Autodesk Inventor part; units mm, degrees
ref_plane "YZ Plane" through (0, 0, 0) normal (1, 0, 0) x (0, 1, 0)
ref_plane "XZ Plane" through (0, 0, 0) normal (0, 1, 0) x (-1, 0, 0)
ref_plane "XY Plane" through (0, 0, 0) normal (0, 0, 1) x (1, 0, 0)
sketch "Sketch1" plane through (0, 0, 0) normal (0, 0, 1) x (1, 0, 0)
  line L0 (-65, 5) -> (65, 5)
  line L1 (65, 5) -> (65, -5)
  line L2 (65, -5) -> (-65, -5)
  line L3 (-65, -5) -> (-65, 5)
  circle A0 centre (0, 0) radius 2.4
  circle A1 centre (-54, 0) radius 2.4
  circle A2 centre (-27, 0) radius 2.4
  circle A3 centre (27, 0) radius 2.4
  circle A4 centre (54, 0) radius 2.4
  line L4 (-65, 0) -> (65, 0) construction
  point P0 (0, 5)
  dimension "d0" = 130
  dimension "d1" = 10
  dimension "d2" = 4.8
  dimension "d3" = 4.8
  dimension "d4" = 4.8
  dimension "d5" = 4.8
  dimension "d6" = 4.8
  dimension "d9" = 27
  dimension "d10" = 27
  dimension "d11" = 27
  dimension "d12" = 27
extrude "Plate1" add sketch "Sketch1" along normal blind 0.5
sketch "Sketch2" plane through (64.5, -5, 0.5) normal (1, 0, 0) x (0, 1, 0)
  line L0 (10, 0) -> (0, 0)
  line L1 (0, 0) -> (0, -5)
  line L2 (0, -5) -> (10, -5)
  line L3 (10, -5) -> (10, 0)
edge flange "Flange1" height 5 angle 90 thickness 0.5 bend radius 0.5 thickness toward (1, 0, 0) relief tear relief width 0.5 relief depth 0.25 corner gap 0.5 corner form 0 edges at (65, 0, 0) (-65, 0, 0) wall of the first edge with corners at (64.5, 5, 0.5) (64.5, -5, 0.5) (64.5, -5, -4.5) (64.5, 5, -4.5)
bend "Bend1"
corner "Corner1"
sketch "Sketch3" plane through (64.5, 5, -4) normal (0, 0, -1) x (-1, 0, 0)
  line L0 (0, -10) -> (0, 0)
  line L1 (0, 0) -> (-7, 0)
  line L2 (-7, 0) -> (-7, -10)
  line L3 (-7, -10) -> (0, -10)
edge flange "Flange2" height 7 angle 90 thickness 0.5 bend radius 0.5 thickness toward (0, 0, -1) relief tear relief width 0.5 relief depth 0.25 corner gap 0.5 corner form 0 edges at (65, 0, -4.5) (-65, 0, -4.5) wall of the first edge with corners at (64.5, -5, -4) (64.5, 5, -4) (71.5, 5, -4) (71.5, -5, -4)
bend "Bend2"
corner "Corner2"
sketch "Sketch4" plane through (-65, -5, -0.5) normal (-1, 0, 0) x (0, 0, 1)
  line L0 (-3, 10) -> (-3, 0)
  line L1 (0, 0) -> (0, 10)
  line L2 (-3, 10) -> (0, 10)
  line L3 (-1.5, 3.5) -> (-1.5, 6.5) construction
  line L4 (-2.5, 3.5) -> (-2.5, 6.5)
  line L5 (-0.5, 6.5) -> (-0.5, 3.5)
  arc A0 (-2.5, 3.5) -> (-0.5, 3.5) centre (-1.5, 3.5) ccw
  arc A1 (-0.5, 6.5) -> (-2.5, 6.5) centre (-1.5, 6.5) ccw
  point P0 (0.5, 5)
  point P1 (-1.5, 5)
  point P2 (-0.5, 5)
  point P3 (0, 5)
  point P4 (-1.5, 7.5)
  point P5 (-1.5, 10)
  dimension "d34" = 2
  dimension "d35" = 5
extrude "Cut1" cut sketch "Sketch4" against normal blind 0.5
mirror "Mirror1" about plane through (0, 0, 0) normal (1, 0, 0) of "Cut1"
equation "\"d36\" = Thickness"
equation "\"d14\" = BendReliefWidth"
equation "\"d15\" = BendReliefDepth"
equation "\"d16\" = MinimumRemnant"
equation "\"d17\" = BendRadius"
equation "\"d20\" = BendRadius"
equation "\"d21\" = CornerReliefSize"
equation "\"d22\" = GapSize"
equation "\"d23\" = JacobiRadiusSize"
equation "\"d24\" = BendReliefWidth"
equation "\"d25\" = BendReliefDepth"
equation "\"d26\" = MinimumRemnant"
equation "\"d27\" = BendRadius"
equation "\"d30\" = BendRadius"
equation "\"d31\" = CornerReliefSize"
equation "\"d32\" = GapSize"
equation "\"d33\" = JacobiRadiusSize"
equation "\"BendRadius\" = Thickness"
equation "\"BendReliefWidth\" = Thickness"
equation "\"BendReliefDepth\" = 0.5 * Thickness"
equation "\"CornerReliefSize\" = 4 * Thickness"
equation "\"MinimumRemnant\" = 2 * Thickness"
equation "\"TransitionRadius\" = BendRadius"
equation "\"JacobiRadiusSize\" = BendRadius"
equation "\"GapSize\" = Thickness"
equation "\"kerf\" = 0.2"
equation "\"d13\" = BendRadius"
properties part number "LEDStripOrigami"
Verification items for the finished model (mm, model axes). A direction names the side the tool comes from. Give positions to 0.01 mm unless a question says otherwise; leave off trailing zeros. Write each loop counter-clockwise with the first axis right and the second up, starting at its lowest first coordinate (ties: lowest second). Pieces come first, ordered by that corner, then holes. Notation, with made-up numbers: M 54.5,1.25 L 66.5,1.25 A30 ccw 66.5,29.25 Z; hole C 66,-38.75 d10. An arc over 180 degrees is marked long. Write item = value, one per line.
(1) Sectioned sample at C-C (x = -22.5). Record the cut outline in (y, z).
Found:
outline = M -5,0 L 5,0 L 5,0.5 L -5,0.5 Z
(2) Sectioned sample at A-A (x = 27). Record the cut outline in (y, z), then the cut area to 3 significant figures.
Found:
outline = M -5,0 L -2.4,0 L -2.4,0.5 L -5,0.5 Z; M 2.4,0 L 5,0 L 5,0.5 L 2.4,0.5 Z
area = 2.60 mm2
(3) Material ranges on line 1 (Y direction, x = 54, z = 0.35); line 2 (X direction, y = -1.5, z = -3.05); line 3 (Z direction, x = 37, y = -2), recorded low to high.
Found:
line_1 = -5 to -2.4, 2.4 to 5
line_2 = -65 to -64.5, 64.5 to 65
line_3 = 0 to 0.5
(4) Sectioned sample at B-B (z = -2). Record the cut outline in (x, y).
Found:
outline = M -65,-5 L -64.5,-5 L -64.5,-2.5 L -65,-2.5 Z; M -65,2.5 L -64.5,2.5 L -64.5,5 L -65,5 Z; M 64.5,-5 L 65,-5 L 65,-2.5 L 64.5,-2.5 Z; M 64.5,2.5 L 65,2.5 L 65,5 L 64.5,5 Z
(5) Go/stop test with flat-tipped pins: pin 1 Ø1.8 at (x, y) = (-70, 1.5) entering from +Z; pin 2 Ø1 at (x, y) = (55.5, 3.5) entering from -Z; pin 3 Ø2.5 at (y, z) = (2, -2) entering from +X. Record where each tip stops, or that it passes through.
Found:
pin_1 = -4
pin_2 = 0
pin_3 = 65
(6) Draft check along X on faces 4 (the face through (65, -0.1, -0.7)), 5 (the face through (68, 0, -4)), 6 (the face through (-24.71, -0.72, 0.25)). Enter one of: released by +X, released by -X, zero draft, split by the parting line, or undercut.
Found:
face_4 = released by +X
face_5 = zero draft
face_6 = undercut
(7) Access from +Z, -Z, +X, -X, +Y, -Y to the whole of each face (thin tool, end or side, straight path). Record for faces 1 (the face through (64.5, -0.07, -0.65)), 2 (the face through (-55.905, 1.46, 0.246)), 3 (the face through (-68, 0, -4)).
Found:
face_1 = -Z, +Y, -Y
face_2 = +Z, -Z
face_3 = +Z, -X, +Y, -Y
